Read the model definition and answer for the solid it produces. Units are mm, in the model's axes. A direction names the side the tool comes from. Round coordinates to 2 decimals unless told otherwise and drop trailing zeros. Loops run counter-clockwise (first coordinate to the right, second up) from the corner with the lowest first, then second, coordinate; pieces in that order, holes last. Notation, with made-up numbers: (75, 6) -> (108, 6) arc R10 cw to (108, 24) -> close; hole circle Ø10 at (67, 9.25). An arc over 180 degrees is marked (long way). Put each result on its own line as item: value.
from build123d import *

# Parameters (mm, degrees)
F0_R        = 2
F0_R_2      = 6.5
F0_W        = 6.35
F0_H        = 44.45
F1_DEPTH    = 5
F2_T1_DEPTH = 28.0247734337
F2_T3_DEPTH = 27.9999173435


# Not quite as in the source:
# - a fillet or chamfer that OpenCascade refuses, or shapes differently, is made with other operations: its cross-section is extruded or revolved along the edge and cut away or added


with BuildPart() as f1:
    # F0 (on Top) → F1 (new body)
    with BuildSketch(Plane.XY):
        with BuildLine():
            Line((-13.2125969287, 28.575), (-15.3026211582, 2.4657221432))
            ThreePointArc((-15.3026211582, 2.4657221432), (0.0013716989, 15.4999999393), (15.3030573351, 2.4630136415))
            Line((15.3030573351, 2.4630136415), (13.2151419082, 28.575))
            Line((13.2151419082, 28.575), (9.4426246963, 28.575))
            Line((9.4426246963, 28.575), (9.4426246963, 75.7550326315))
            ThreePointArc((9.4426246963, 75.7550326315), (-0.1780593733, 84.4710891818), (-9.464331693, 75.3995760688))
            Line((-9.464331693, 75.3995760688), (-9.464331693, 28.575))
            Line((-9.464331693, 28.575), (-13.2125969287, 28.575))
        make_face()
        Polygon((6.35, 73.025), (6.35, 28.575), (3.175, 28.575), (-3.175, 28.575), (-6.35, 28.575), (-6.35, 73.025), (-3.175, 73.025), (3.175, 73.025), align=None, mode=Mode.SUBTRACT)
        with BuildLine():
            Line((-15.3026211582, 2.4657221432), (-15.5, 0))
            ThreePointArc((-15.5, 0), (0, -15.5), (15.5, 0))
            Line((15.5, 0), (15.3030573351, 2.4630136415))
            ThreePointArc((15.3030573351, 2.4630136415), (0.0013716989, 15.4999999393), (-15.3026211582, 2.4657221432))
        make_face()
        with Locations((-9.9, 0)):
            Circle(F0_R, mode=Mode.SUBTRACT)
        with Locations((0, -9.9)):
            Circle(F0_R, mode=Mode.SUBTRACT)
        Circle(F0_R_2, mode=Mode.SUBTRACT)
        with Locations((9.9, 0)):
            Circle(F0_R, mode=Mode.SUBTRACT)
        with Locations((0, 9.9)):
            Circle(F0_R, mode=Mode.SUBTRACT)
        with Locations((0, 50.8)):
            Rectangle(F0_W, F0_H)
    extrude(amount=F1_DEPTH)

    # F2: fillet of radius 5.08 on 2 edges, made by hand

    # F2_s2 → F2_t1 (cut)
    with BuildSketch(Plane.XY.offset(-11.5123867168)):
        with BuildLine():
            ThreePointArc((13.5821827728, 23.9846962333), (12.2908918839, 26.9818924846), (9.4426246963, 28.575))
            Line((9.4426246963, 28.575), (13.2151419082, 28.575))
            Line((13.2151419082, 28.575), (13.5821827728, 23.9846962333))
        make_face()
    extrude(amount=F2_T1_DEPTH, mode=Mode.SUBTRACT)

    # F2_s4 → F2_t3 (cut)
    with BuildSketch(Plane.XY.offset(-11.4999586717)):
        with BuildLine():
            ThreePointArc((-9.464331693, 28.575), (-12.2964780323, 26.9774445837), (-13.579647346, 23.9896840999))
            Line((-13.579647346, 23.9896840999), (-13.2125969287, 28.575))
            Line((-13.2125969287, 28.575), (-9.464331693, 28.575))
        make_face()
    extrude(amount=F2_T3_DEPTH, mode=Mode.SUBTRACT)


solid = f1.part
Item 1: For a pull along X with two mould halves and no side action, classify faces 1 (the flat face through (-9.464, 52, 2)), 2 (the cylindrical face through (0.923, -11.674, 2.465)), 3 (the flat face through (9.443, 52, 2)), 4 (the flat face through (3.175, 50, 2)) as pulls with the +X half, pulls with the -X half, needs draft (parallel to the pull), parting line crosses it, or undercut.
Derived:
face 1: pulls with the -X half
face 2: undercut
face 3: pulls with the +X half
face 4: undercut
Item 2: The part is cut by section A-A (y = 71.5). Determine the outline of the cut face in (x, z) (3 decimals).
Derived:
outline: (-9.464, 0) -> (-6.35, 0) -> (-6.35, 5) -> (-9.464, 5) -> close; (-3.175, 0) -> (3.175, 0) -> (3.175, 5) -> (-3.175, 5) -> close; (6.35, 0) -> (9.443, 0) -> (9.443, 5) -> (6.35, 5) -> close
Item 3: Which of the six approach directions +Z, -Z, +X, -X, +Y, -Y give full straight-line access (tool end or side, diameter ignored) to faces 5 (the flat face through (-6.35, 50, 2)), 6 (the cylindrical face through (0.022, 84.473, 2.465))?
Derived:
face 5: +Z, -Z
face 6: +Z, -Z, +Y
Item 4: The part is cut by section B-B (x = 0). Determine the outline of the cut face in (y, z), then the cut area to 3 significant figures.
Derived:
outline: (-15.5, 0) -> (-11.9, 0) -> (-11.9, 5) -> (-15.5, 5) -> close; (-7.9, 0) -> (-6.5, 0) -> (-6.5, 5) -> (-7.9, 5) -> close; (6.5, 0) -> (7.9, 0) -> (7.9, 5) -> (6.5, 5) -> close; (11.9, 0) -> (84.47, 0) -> (84.47, 5) -> (11.9, 5) -> close
area: 395 mm^2
Item 5: Find the intervals of material crossed by line 1 along Y through (x, z) = (0, 3.2); line 2 along X through (y, z) = (38.5, 4.7) (3 decimals); line 3 along Y through (x, z) = (-0.5, 0.8), in increasing order.
Derived:
line 1: y = -15.5 to -11.9, -7.9 to -6.5, 6.5 to 7.9, 11.9 to 84.47
line 2: x = -9.464 to -6.35, -3.175 to 3.175, 6.35 to 9.443
line 3: y = -15.49 to -11.84, -7.96 to -6.48, 6.48 to 7.96, 11.84 to 84.46
Item 6: The part is cut by section D-D (y = 1). Determine the outline of the cut face in (x, z), then the cut area to 3 significant figures.
Derived:
outline: (-15.42, 0) -> (-11.63, 0) -> (-11.63, 5) -> (-15.42, 5) -> close; (-8.17, 0) -> (-6.42, 0) -> (-6.42, 5) -> (-8.17, 5) -> close; (6.42, 0) -> (8.17, 0) -> (8.17, 5) -> (6.42, 5) -> close; (11.63, 0) -> (15.42, 0) -> (15.42, 5) -> (11.63, 5) -> close
area: 55.3 mm^2
Item 7: The part is cut by section C-C (z = 4.2). Determine the outline of the cut face in (x, y) (3 decimals), then the cut area to 3 significant figures.
Derived:
outline: (-15.5, 0) arc R15.5 ccw to (15.5, 0) -> (13.582, 23.985) arc R5.08 ccw to (9.443, 28.575) -> (9.443, 75.755) arc R9.473 ccw to (-9.464, 75.4) -> (-9.464, 28.575) arc R5.08 ccw to (-13.58, 23.99) -> close; hole circle Ø4 at (-9.9, 0); hole circle Ø13 at (0, 0); hole (-6.35, 28.575) -> (-3.175, 28.575) -> (-3.175, 73.025) -> (-6.35, 73.025) -> close; hole circle Ø4 at (0, -9.9); hole circle Ø4 at (0, 9.9); hole (3.175, 28.575) -> (6.35, 28.575) -> (6.35, 73.025) -> (3.175, 73.025) -> close; hole circle Ø4 at (9.9, 0)
area: 1,740 mm^2
Item 8: Flat-ended cylindrical pins translate along their axes: pin 1 Ø1 at (x, z) = (-3.5, 3) entering from +Y; pin 2 Ø1.5 at (y, z) = (63.5, 1.5) entering from +X; pin 3 Ø1.6 at (x, z) = (5.5, 2.5) entering from -Y. Find the tip coordinate at first contact, or state that the pin passes through.
Derived:
pin 1: stops at y = 83.99
pin 2: stops at x = 9.44
pin 3: stops at y = -14.77
